```python
from build123d import *

# Parameters (mm, degrees)
F1_DEPTH = 19.05
F4_DEPTH = 19.051
F6_DEPTH = 19.051
F7_DEPTH = 19.051


with BuildPart() as f1:
    # F0 (on Front) → F1 (new body)
    with BuildSketch(Plane.XZ):
        with BuildLine():
            ThreePointArc((7.08977, 74.735215), (-4.612113, 72.936745), (-10.446423, 62.634833))
            ThreePointArc((-10.446423, 62.634833), (-45.232522, 44.567577), (-62.782662, 9.51774))
            ThreePointArc((-62.782662, 9.51774), (-63.498259, -0.470187), (-62.634833, -10.446423))
            ThreePointArc((-62.634833, -10.446423), (-44.567577, -45.232522), (-9.51774, -62.782662))
            ThreePointArc((-9.51774, -62.782662), (0.470187, -63.498259), (10.446423, -62.634833))
            ThreePointArc((10.446423, -62.634833), (45.232522, -44.567577), (62.782662, -9.51774))
            ThreePointArc((62.782662, -9.51774), (63.498259, 0.470187), (62.634833, 10.446423))
            ThreePointArc((62.634833, 10.446423), (44.567577, 45.232522), (9.51774, 62.782662))
            ThreePointArc((9.51774, 62.782662), (4.127105, 67.910519), (7.08977, 74.735215))
        make_face()
        with BuildLine():
            ThreePointArc((-62.634833, -10.446423), (-63.498259, -0.470187), (-62.782662, 9.51774))
            ThreePointArc((-62.782662, 9.51774), (-67.910519, 4.127105), (-74.735215, 7.08977))
            ThreePointArc((-74.735215, 7.08977), (-72.936745, -4.612113), (-62.634833, -10.446423))
        make_face()
        with BuildLine():
            ThreePointArc((74.735215, -7.08977), (72.936745, 4.612113), (62.634833, 10.446423))
            ThreePointArc((62.634833, 10.446423), (63.498259, 0.470187), (62.782662, -9.51774))
            ThreePointArc((62.782662, -9.51774), (67.910519, -4.127105), (74.735215, -7.08977))
        make_face()
        with BuildLine():
            ThreePointArc((10.446423, -62.634833), (0.470187, -63.498259), (-9.51774, -62.782662))
            ThreePointArc((-9.51774, -62.782662), (-4.127105, -67.910519), (-7.08977, -74.735215))
            ThreePointArc((-7.08977, -74.735215), (4.612113, -72.936745), (10.446423, -62.634833))
        make_face()
    extrude(amount=F1_DEPTH)

    # F3 (on face) → F4 (cut, through all)
    with BuildSketch(Plane.XZ.offset(19.05)):
        with BuildLine():
            Line((39.873943, 79.150751), (9.51774, 62.782662))
            ThreePointArc((9.51774, 62.782662), (23.239874, 23.586611), (62.634833, 10.446423))
            Line((62.634833, 10.446423), (86.088315, 35.227999))
            Line((86.088315, 35.227999), (39.873943, 79.150751))
        make_face()
        with BuildLine():
            Line((-79.150751, 39.873943), (-62.782662, 9.51774))
            ThreePointArc((-62.782662, 9.51774), (-23.586611, 23.239874), (-10.446423, 62.634833))
            Line((-10.446423, 62.634833), (-35.227999, 86.088315))
            Line((-35.227999, 86.088315), (-79.150751, 39.873943))
        make_face()
        with BuildLine():
            Line((-39.873943, -79.150751), (-9.51774, -62.782662))
            ThreePointArc((-9.51774, -62.782662), (-23.239874, -23.586611), (-62.634833, -10.446423))
            Line((-62.634833, -10.446423), (-86.088315, -35.227999))
            Line((-86.088315, -35.227999), (-39.873943, -79.150751))
        make_face()
        with BuildLine():
            Line((79.150751, -39.873943), (62.782662, -9.51774))
            ThreePointArc((62.782662, -9.51774), (23.586611, -23.239874), (10.446423, -62.634833))
            Line((10.446423, -62.634833), (35.227999, -86.088315))
            Line((35.227999, -86.088315), (79.150751, -39.873943))
        make_face()
    extrude(amount=-F4_DEPTH, mode=Mode.SUBTRACT)

    # F5 (on face) → F6 (cut, through all)
    with BuildSketch(Plane.XZ.offset(19.05)):
        with BuildLine():
            ThreePointArc((-5.122292, 49.557197), (0, 44.457518), (5.122292, 49.557197))
            ThreePointArc((5.122292, 49.557197), (3.175, 53.635843), (5.122292, 57.714488))
            Line((5.122292, 57.714488), (9.185783, 57.714488))
            ThreePointArc((9.185783, 57.714488), (9.283466, 60.253048), (9.51774, 62.782662))
            ThreePointArc((9.51774, 62.782662), (4.127105, 67.910519), (7.08977, 74.735215))
            ThreePointArc((7.08977, 74.735215), (-4.612113, 72.936745), (-10.446423, 62.634833))
            ThreePointArc((-10.446423, 62.634833), (-10.180474, 60.179939), (-10.043413, 57.714488))
            Line((-10.043413, 57.714488), (-5.122292, 57.714488))
            ThreePointArc((-5.122292, 57.714488), (-3.175, 53.635843), (-5.122292, 49.557197))
        make_face()
        with BuildLine():
            Line((-57.714488, 5.122292), (-57.714488, 9.185783))
            ThreePointArc((-57.714488, 9.185783), (-60.253048, 9.283466), (-62.782662, 9.51774))
            ThreePointArc((-62.782662, 9.51774), (-67.910519, 4.127105), (-74.735215, 7.08977))
            ThreePointArc((-74.735215, 7.08977), (-72.936745, -4.612113), (-62.634833, -10.446423))
            ThreePointArc((-62.634833, -10.446423), (-60.179939, -10.180474), (-57.714488, -10.043413))
            Line((-57.714488, -10.043413), (-57.714488, -5.122292))
            ThreePointArc((-57.714488, -5.122292), (-53.635843, -3.175), (-49.557197, -5.122292))
            ThreePointArc((-49.557197, -5.122292), (-44.457518, 0), (-49.557197, 5.122292))
            ThreePointArc((-49.557197, 5.122292), (-53.635843, 3.175), (-57.714488, 5.122292))
        make_face()
        with BuildLine():
            ThreePointArc((10.446423, -62.634833), (10.180474, -60.179939), (10.043413, -57.714488))
            Line((10.043413, -57.714488), (5.122292, -57.714488))
            ThreePointArc((5.122292, -57.714488), (3.175, -53.635843), (5.122292, -49.557197))
            ThreePointArc((5.122292, -49.557197), (0, -44.457518), (-5.122292, -49.557197))
            ThreePointArc((-5.122292, -49.557197), (-3.175, -53.635843), (-5.122292, -57.714488))
            Line((-5.122292, -57.714488), (-9.185783, -57.714488))
            ThreePointArc((-9.185783, -57.714488), (-9.283466, -60.253048), (-9.51774, -62.782662))
            ThreePointArc((-9.51774, -62.782662), (-4.127105, -67.910519), (-7.08977, -74.735215))
            ThreePointArc((-7.08977, -74.735215), (4.612113, -72.936745), (10.446423, -62.634833))
        make_face()
        with BuildLine():
            ThreePointArc((62.634833, 10.446423), (60.179939, 10.180474), (57.714488, 10.043413))
            Line((57.714488, 10.043413), (57.714488, 5.122292))
            ThreePointArc((57.714488, 5.122292), (53.635843, 3.175), (49.557197, 5.122292))
            ThreePointArc((49.557197, 5.122292), (44.457518, 0), (49.557197, -5.122292))
            ThreePointArc((49.557197, -5.122292), (53.635843, -3.175), (57.714488, -5.122292))
            Line((57.714488, -5.122292), (57.714488, -9.185783))
            ThreePointArc((57.714488, -9.185783), (60.253048, -9.283466), (62.782662, -9.51774))
            ThreePointArc((62.782662, -9.51774), (67.910519, -4.127105), (74.735215, -7.08977))
            ThreePointArc((74.735215, -7.08977), (72.936745, 4.612113), (62.634833, 10.446423))
        make_face()
    extrude(amount=-F6_DEPTH, mode=Mode.SUBTRACT)

    # F2 (on face) → F7 (cut, through all)
    with BuildSketch(Plane(origin=(0, 0, 0), x_dir=(-1, 0, 0), z_dir=(0, 1, 0))):
        with BuildLine():
            Line((-1.5875, 1.5875), (-2.601951, 1.5875))
            ThreePointArc((-2.601951, 1.5875), (0, -3.048), (2.601951, 1.5875))
            Line((2.601951, 1.5875), (-1.5875, 1.5875))
        make_face()
    extrude(amount=-F7_DEPTH, mode=Mode.SUBTRACT)


solid = f1.part
```
The listing builds one solid part. Answer for the finished solid, in the listing's coordinates (mm). A direction names the side the tool comes from. Coordinates: 2 decimals unless noted, no trailing zeros. Write each loop counter-clockwise with the first axis right and the second up, starting at its lowest first coordinate (ties: lowest second). Pieces come first, ordered by that corner, then holes. Notation, with made-up numbers: (50.25, 7.5) - (97.25, 7.5) arc R16 ccw to (97.25, 37.5) - close; hole circle Ø4 at (-21, 74.5). An arc over 180 degrees is marked (long way). Return JSON: item names as keys, results as strings. Group by question number.
1. A cutting plane is placed at A-A, the plane y = -1.75. Determine the outline of the cut face in (x, z), plus the area to 3 significant figures.
2. A cutting plane is placed at D-D, the plane z = -20.5. Determine the outline of the cut face in (x, y), plus the area to 3 significant figures.
3. Straight lines are drawn through the part: L1, parallel to Z at x = 0, y = -8; L2, parallel to X at y = -4.75, z = 0; L3, parallel to Z at x = -51, y = -2.5. For each, find the intervals that lie inside material, in ascending order.
4. Determine the mould class of faces 3 (the flat face through (8, -10, -57.714)), 4 (the flat face through (57.714, -10, 8)), 5 (the cylindrical face through (0.09, -9.392, -3.047)) for opening direction X: released by +X, released by -X, zero draft, split by the parting line, or undercut.
5. Given pin 1 (10 mm diameter, centred on x = 40.5, y = -11.5, fed in from +Z); pin 2 (6 mm diameter, centred on x = -23.5, y = -13.5, fed in from -Z); pin 3 (10 mm diameter, centred on y = -4.5, z = -20.5, fed in from +X), each flat-ended and moving along its own axis, determine where each tip first touches the part or whether it passes through.
6. A cutting plane is placed at C-C, the plane x = 0. Determine the outline of the cut face in (y, z).
7. Which of the six approach directions +Z, -Z, +X, -X, +Y, -Y give full straight-line access (tool end or side, diameter ignored) to faces 1 (the cylindrical face through (-3.175, -9.658, 53.701)), 2 (the flat face through (7, -10, 57.714))?
8. A cutting plane is placed at B-B, the plane z = 0. Determine the outline of the cut face in (x, y).
Ans:
{
 "1": {"outline": "(-57.71, -10.04) arc R47.15 cw to (-9.19, -57.71) - (-5.12, -57.71) arc R5.25 ccw to (-5.12, -49.56) arc R5.12 cw to (5.12, -49.56) arc R5.25 ccw to (5.12, -57.71) - (10.04, -57.71) arc R47.15 cw to (57.71, -9.19) - (57.71, -5.12) arc R5.25 ccw to (49.56, -5.12) arc R5.12 cw to (49.56, 5.12) arc R5.25 ccw to (57.71, 5.12) - (57.71, 10.04) arc R47.15 cw to (9.19, 57.71) - (5.12, 57.71) arc R5.25 ccw to (5.12, 49.56) arc R5.12 cw to (-5.12, 49.56) arc R5.25 ccw to (-5.12, 57.71) - (-10.04, 57.71) arc R47.15 cw to (-57.71, 9.19) - (-57.71, 5.12) arc R5.25 ccw to (-49.56, 5.12) arc R5.12 cw to (-49.56, -5.12) arc R5.25 ccw to (-57.71, -5.12) - close; hole (-2.6, 1.59) arc R3.05 ccw (long way) to (2.6, 1.59) - close", "area": "5,540 mm²"},
 "2": {"outline": "(-26.7, -19.05) - (26.53, -19.05) - (26.53, 0) - (-26.7, 0) - close", "area": "1,010 mm²"},
 "3": {"L1": "-44.46 to -3.05, 1.59 to 44.46", "L2": "-44.46 to -3.05, 3.05 to 44.46", "L3": "-10.33 to -3.89, 3.89 to 9.59"},
 "4": {"face 3": "zero draft", "face 4": "released by +X", "face 5": "undercut"},
 "5": {"pin 1": "z = 14.87", "pin 2": "z = -26.53", "pin 3": "x = 33.6"},
 "6": {"outline": "(-19.05, -44.46) - (0, -44.46) - (0, -3.05) - (-19.05, -3.05) - close; (-19.05, 1.59) - (0, 1.59) - (0, 44.46) - (-19.05, 44.46) - close"},
 "7": {"face 1": "+Y, -Y", "face 2": "+Z, +X, -X, +Y, -Y"},
 "8": {"outline": "(-44.46, -19.05) - (-3.05, -19.05) - (-3.05, 0) - (-44.46, 0) - close; (3.05, -19.05) - (44.46, -19.05) - (44.46, 0) - (3.05, 0) - close"}
}
